Can you work these out from the model? Positions are in its coordinate system, mm. Face numbers are marked on the shaded views. A direction names the side the tool comes from. Coordinates: 2 decimals unless noted, no trailing zeros. Order: outer loops, then holes, each group sorted by start corner. A loop starts at its lowest first (then second) coordinate and runs counter-clockwise, first axis right, second up. Notation, with made-up numbers: (-39.5, 10) - (-19.5, 10) arc R13 cw to (-19.5, 15) - close; hole circle Ø1 at (44.5, 15.5). An arc over 180 degrees is marked (long way). Return JSON: item names as keys, results as strings. Group by question number.
1) If I drill on line 1 along Y through (x, z) = (-68, -27.05); line 2 along Y through (x, z) = (-76.5, -25.5); line 3 along Z through (x, y) = (-68.25, -4.5), over which ranges is the centre line in solid material (lowest first)?
2) Imagine slicing it at C-C (x = -81.5). Write out the boundary of the cut face in (y, z).
3) Imagine slicing it at B-B (y = 15.5). Write out the boundary of the cut face in (x, z).
4) Which directions (+Z, -Z, +X, -X, +Y, -Y) give clear straight access to the entire face, cutting with the end or side of a thin tool? Please do the marked faces 1, 2 and 3.
5) Imagine slicing it at D-D (z = -26.15). Write out the boundary of the cut face in (x, y).
6) For pin 1 Ø1 at (y, z) = (4.5, -26) entering from +X; pin 2 Ø2 at (x, z) = (-73.5, -27) entering from -Y; pin 3 Ø1.5 at (y, z) = (3, -26.5) entering from -X, each with a flat end and sliding along its axis, tell me the tip position at first contact or that it passes through.
7) Imagine slicing it at A-A (z = -28). Write out the boundary of the cut face in (x, y).
```python
from build123d import *

# Parameters (mm, degrees)
BOSS_EXTRUDE5_DEPTH = 2
SKETCH5_R           = 2
BOSS_EXTRUDE6_DEPTH = 25
BOSS_EXTRUDE7_START = 12
SKETCH6_R           = 1.5
BOSS_EXTRUDE7_DEPTH = 12


with BuildPart() as part:
    # Sketch1 → Boss-Extrude5 (new body)
    with BuildSketch(Plane(origin=(0, 0, 0), x_dir=(1, 0, 0), z_dir=(0, 1, 0))):
        with BuildLine():
            Line((-80.770804267, 29.795413952), (-68.129526639, 28.795413952))
            ThreePointArc((-68.129526639, 28.795413952), (-66.629526639, 27.295413952), (-68.129526639, 25.795413952))
            Line((-68.129526639, 25.795413952), (-80.770804267, 24.795413952))
            ThreePointArc((-80.770804267, 24.795413952), (-83.270804267, 27.295413952), (-80.770804267, 29.795413952))
        make_face()
    extrude(amount=BOSS_EXTRUDE5_DEPTH)

    # Sketch5 → Boss-Extrude6 (add)
    with BuildSketch(Plane(origin=(0, 2, 0), x_dir=(1, 0, 0), z_dir=(0, 1, 0))):
        with Locations(Location((-80.770804267, 27.295413952, 0), (0, 0, 270))):
            Circle(SKETCH5_R)
    extrude(amount=BOSS_EXTRUDE6_DEPTH)

    # Sketch6 → Boss-Extrude7 (add)
    with BuildSketch(Plane.XZ.offset(BOSS_EXTRUDE7_START)):
        with Locations(Location((-68.129526639, -27.295413952, 0), (0, 0, 270))):
            Circle(SKETCH6_R)
    extrude(amount=-BOSS_EXTRUDE7_DEPTH)


solid = part.part
```
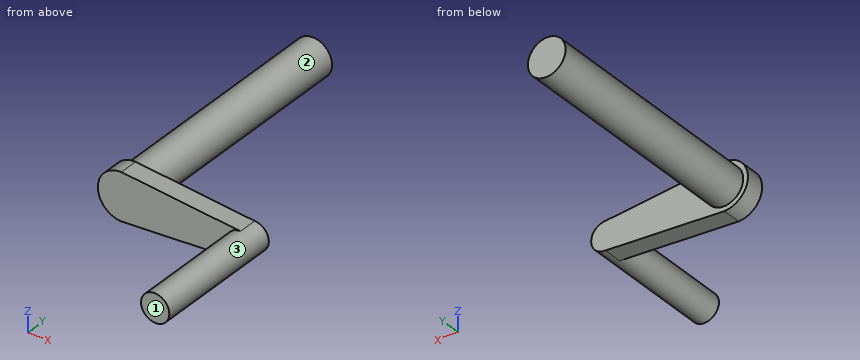
Calculated:
{
 "1": {"line 1": "-12 to 2", "line 2": "0 to 2", "line 3": "-28.79 to -25.8"},
 "2": {"outline": "(0, -29.69) - (2, -29.69) - (2, -29.16) - (27, -29.16) - (27, -25.43) - (2, -25.43) - (2, -24.9) - (0, -24.9) - close"},
 "3": {"outline": "circle Ø4 at (-80.77, -27.3)"},
 "4": {"face 1": "+Z, -Z, +X, -X, -Y", "face 2": "+Y", "face 3": "-Y"},
 "5": {"outline": "(-82.99, 0) - (-69.1, 0) - (-69.1, -12) - (-67.16, -12) - (-67.16, 2) - (-79.13, 2) - (-79.13, 27) - (-82.41, 27) - (-82.41, 2) - (-82.99, 2) - close"},
 "6": {"pin 1": "x = -78.94", "pin 2": "y = 0", "pin 3": "x = -82.77"},
 "7": {"outline": "(-83.17, 0) - (-69.45, 0) - (-69.45, -12) - (-66.81, -12) - (-66.81, 2) - (-78.9, 2) - (-78.9, 27) - (-82.64, 27) - (-82.64, 2) - (-83.17, 2) - close"}
}
